```python
from build123d import *

# Parameters (mm, degrees)
CROQUIS3_W              = 50.8
CROQUIS3_H              = 25.4
CROQUIS3_R              = 3.175
SALIENTE_EXTRUIR1_DEPTH = 3.175
CROQUIS6_R              = 0.762
SALIENTE_EXTRUIR3_DEPTH = 8.466666667


with BuildPart() as part:
    # Croquis3 → Saliente-Extruir1 (new body)
    with BuildSketch(Plane(origin=(0, 0, 0), x_dir=(1, 0, 0), z_dir=(0, 1, 0))):
        Rectangle(CROQUIS3_W, CROQUIS3_H)
        with Locations((-12.7, 0)):
            Circle(CROQUIS3_R, mode=Mode.SUBTRACT)
        with Locations((12.7, 0)):
            Circle(CROQUIS3_R, mode=Mode.SUBTRACT)
    extrude(amount=SALIENTE_EXTRUIR1_DEPTH)

    # Croquis6 → Saliente-Extruir3 (add, symmetric)
    with BuildSketch(Plane.ZY):
        with BuildLine():
            Line((-12.7, 3.175), (-13.208, 3.175))
            Line((-13.208, 3.175), (-13.208, 2.437497499))
            ThreePointArc((-13.208, 2.437497499), (-13.301057822, 2.315117237), (-13.443857143, 2.372082497))
            ThreePointArc((-13.443857143, 2.372082497), (-16.51, 1.521687475), (-13.443857143, 0.671292453))
            ThreePointArc((-13.443857143, 0.671292453), (-13.301057822, 0.728257713), (-13.208, 0.605877451))
            Line((-13.208, 0.605877451), (-13.208, 0))
            Line((-13.208, 0), (-12.7, 0))
            Line((-12.7, 0), (-12.7, 3.175))
        make_face()
        with Locations((-14.859, 1.521687475)):
            Circle(CROQUIS6_R, mode=Mode.SUBTRACT)
    extrude(amount=SALIENTE_EXTRUIR3_DEPTH, both=True)


solid = part.part
```
Geometry check sheet. Reference: the model listing, model coordinates, mm. A direction names the side the tool comes from. Give positions to 0.01 mm unless a question says otherwise; leave off trailing zeros. Write each loop counter-clockwise with the first axis right and the second up, starting at its lowest first coordinate (ties: lowest second). Pieces come first, ordered by that corner, then holes. Notation, with made-up numbers: (24, 57) -> (57, 57) arc R16 ccw to (57, 79) -> close; hole circle Ø1 at (71.5, 42.25). An arc over 180 degrees is marked (long way). Use one line per item in the form item = value.
Item 1: Sectioned sample at D-D on z = -7.5. Enter the section's corners in (x, y) (3 decimals), plus the area to 3 significant figures.
Results list:
outline = (-25.4, 0) -> (25.4, 0) -> (25.4, 3.175) -> (-25.4, 3.175) -> close
area = 161 mm2
Item 2: Mould release check, pull along X, two halves, no side actions. Record for faces 1 (the flat face through (8.467, 2, -14)), 2 (the cylindrical face through (-0.12, 1.58, -16.51)), 3 (the cylindrical face through (-9.67, 1.57, -0.95)), 4 (the cylindrical face through (9.53, 1.57, -0.14)): released by +X, released by -X, zero draft, split by the parting line, or undercut.
Results list:
face_1 = released by +X
face_2 = zero draft
face_3 = undercut
face_4 = undercut
Item 3: Depth check by flat-ended pin: pin 1 Ø1 at (x, y) = (-19, 2) entering from -Z; pin 2 Ø0.6 at (x, y) = (2.5, 3) entering from -Z; pin 3 Ø7.5 at (x, z) = (-12.7, 0) entering from -Y. Enter the tip coordinate at first touch or a pass-through.
Results list:
pin_1 = -12.7
pin_2 = -16.02
pin_3 = 0
Item 4: Sectioned sample at A-A on z = 0. Enter the section's corners in (x, y) (3 decimals), plus the area to 3 significant figures.
Results list:
outline = (-25.4, 0) -> (-15.875, 0) -> (-15.875, 3.175) -> (-25.4, 3.175) -> close; (-9.525, 0) -> (9.525, 0) -> (9.525, 3.175) -> (-9.525, 3.175) -> close; (15.875, 0) -> (25.4, 0) -> (25.4, 3.175) -> (15.875, 3.175) -> close
area = 121 mm2
Item 5: Access from +Z, -Z, +X, -X, +Y, -Y to the whole of each face (thin tool, end or side, straight path). Record for faces 5 (the flat face through (-17, 2, -12.7)), 6 (the flat face through (17, 2, -12.7)), 7 (the flat face through (25.4, 2, 0)), 8 (the flat face through (0, 0, 0)).
Results list:
face_5 = -Z, -X, +Y, -Y
face_6 = -Z, +X, +Y, -Y
face_7 = +Z, -Z, +X, +Y, -Y
face_8 = +Z, +X, -X, -Y
Item 6: Sectioned sample at B-B on x = 12.7. Enter the section's corners in (y, z) (3 decimals).
Results list:
outline = (0, -12.7) -> (3.175, -12.7) -> (3.175, -3.175) -> (0, -3.175) -> close; (0, 3.175) -> (3.175, 3.175) -> (3.175, 12.7) -> (0, 12.7) -> close
Item 7: Scan lines: line 1 (X direction, y = 1.7, z = 0) (3 decimals); line 2 (Z direction, x = -12.7, y = 2) (3 decimals); line 3 (X direction, y = 0.6, z = -0.75). Record each from-to range of solid material in increasing order.
Results list:
line_1 = -25.4 to -15.875, -9.525 to 9.525, 15.875 to 25.4
line_2 = -12.7 to -3.175, 3.175 to 12.7
line_3 = -25.4 to -15.79, -9.61 to 9.61, 15.79 to 25.4
